from build123d import *

# Parameters (mm, degrees)
WALL_DEPTH                = 19.05
ROOF_START                = 19.05
ROOF_DEPTH                = 3.175
F_2_56_TAPPED_HOLE1_D     = 1.778
F_2_56_TAPPED_HOLE1_DEPTH = 5.73
F_2_56_TAPPED_HOLE1_TIP   = 0.53416509


with BuildPart() as part:
    # MainSketch → Wall (new body)
    with BuildSketch(Plane(origin=(0, 0, 0), x_dir=(1, 0, 0), z_dir=(0, 1, 0))):
        Polygon((-32.75, -4), (0, -4), (0, 0), (-36.75, 0), (-36.75, -45.5), (0, -45.5), (0, -41.5), (-32.75, -41.5), align=None)
    extrude(amount=WALL_DEPTH)

    # MainSketch<3> → Roof (add)
    with BuildSketch(Plane(origin=(0, 0, 0), x_dir=(1, 0, 0), z_dir=(0, 1, 0)).offset(ROOF_START)):
        with BuildLine():
            Line((0, -21.625), (0, 0))
            Line((0, 0), (-36.75, 0))
            Line((-36.75, 0), (-36.75, -45.5))
            Line((-36.75, -45.5), (0, -45.5))
            Line((0, -45.5), (0, -23.875))
            ThreePointArc((0, -23.875), (-0.353553391, -23.728553391), (-0.5, -23.375))
            Line((-0.5, -23.375), (-0.5, -22.125))
            ThreePointArc((-0.5, -22.125), (-0.353553391, -21.771446609), (0, -21.625))
        make_face()
    extrude(amount=ROOF_DEPTH)

    # #2-56 Tapped Hole1
    with Locations(Plane(origin=(-10, 0, 43), x_dir=(0, 0, -1), z_dir=(0, -1, 0))):
        with Locations((0, 0), (0, -24.25), (40.5, -24.25), (40.5, 0)):
            Hole(F_2_56_TAPPED_HOLE1_D / 2, depth=F_2_56_TAPPED_HOLE1_DEPTH)
            with Locations((0, 0, -(F_2_56_TAPPED_HOLE1_DEPTH + F_2_56_TAPPED_HOLE1_TIP / 2))):  # 118° drill point
                Cone(0, F_2_56_TAPPED_HOLE1_D / 2, F_2_56_TAPPED_HOLE1_TIP, mode=Mode.SUBTRACT)


solid = part.part
The listing builds one solid part. Answer for the finished solid, in the listing's coordinates (mm). A direction names the side the tool comes from. Round coordinates to 2 decimals unless told otherwise and drop trailing zeros. Order: outer loops, then holes, each group sorted by start corner. A loop starts at its lowest first (then second) coordinate and runs counter-clockwise, first axis right, second up. Notation, with made-up numbers: M 71.5,79.25 L 102.5,79.25 A33 ccw 102.5,117.25 Z; hole C 26.5,56.5 d4. An arc over 180 degrees is marked long. Answer in a Markdown table with one row per item. Add a question column.
1) The part is cut by section D-D on z = 20. Determine the outline of the cut face in (x, y) (3 decimals), plus the area to 3 significant figures.
2) Which of the six approach directions +Z, -Z, +X, -X, +Y, -Y give full straight-line access (tool end or side, diameter ignored) to faces 1 (the face through (-17, 19.05, 22)), 2 (the face through (-9.12, 2.91, 2.38)), 3 (the face through (-18, 11, 0))?
3) Consider line 1 along Z through (x, y) = (-10, 2.1); line 2 along X through (y, z) = (2.2, 43); line 3 along Z through (x, y) = (-34.25, 4). Determine where each line is inside the solid, lowest interval first. Write a range as from..to.
4) The part is cut by section B-B on x = -20. Determine the outline of the cut face in (y, z) (3 decimals).
5) The part is cut by section A-A on y = 3. Determine the outline of the cut face in (x, z), plus the area to 3 significant figures.
6) Flat-ended cylindrical pins translate along their axes: pin 1 Ø1.6 at (x, z) = (-34.25, 2.5) entering from -Y; pin 2 Ø0.6 at (y, z) = (20.5, 22.5) entering from +X; pin 3 Ø6 at (y, z) = (4, 14) entering from +X. Find the tip coordinate at first contact, or state that the pin passes through.
7) Determine the mould class of faces 4 (the face through (0, 14.4, 3.7)), 5 (the face through (-9.847, 6.171, 2.52)), 6 (the face through (-33, 0, 23)) for opening direction X: pulls with the +X half, pulls with the -X half, needs draft (parallel to the pull), parting line crosses it, or undercut.
8) The part is cut by section C-C on y = 12.25. Determine the outline of the cut face in (x, z), plus the area to 3 significant figures.
Findings below:
| question | item | result |
|---|---|---|
| 1 | outline | M -36.75,0 L -32.75,0 L -32.75,19.05 L 0,19.05 L 0,22.225 L -36.75,22.225 Z |
| 1 | area | 193 mm² |
| 2 | face 1 | +X, -Y |
| 2 | face 2 | -Y |
| 2 | face 3 | -Z, +X, -X, +Y, -Y |
| 3 | line 1 | z = 0..1.61, 3.39..4, 41.5..42.11, 43.89..45.5 |
| 3 | line 2 | x = -36.75..-35.14, -33.36..-10.89, -9.11..0 |
| 3 | line 3 | z = 0..1.61, 3.39..42.11, 43.89..45.5 |
| 4 | outline | M 0,0 L 22.225,0 L 22.225,45.5 L 0,45.5 L 0,41.5 L 19.05,41.5 L 19.05,4 L 0,4 Z |
| 5 | outline | M -36.75,0 L 0,0 L 0,4 L -32.75,4 L -32.75,41.5 L 0,41.5 L 0,45.5 L -36.75,45.5 Z; hole C -34.25,2.5 d1.78; hole C -34.25,43 d1.78; hole C -10,2.5 d1.78; hole C -10,43 d1.78 |
| 5 | area | 434 mm² |
| 6 | pin 1 | stops at y = 5.78 |
| 6 | pin 2 | stops at x = -0.5 |
| 6 | pin 3 | stops at x = -32.75 |
| 7 | face 4 | pulls with the +X half |
| 7 | face 5 | undercut |
| 7 | face 6 | needs draft |
| 8 | outline | M -36.75,0 L 0,0 L 0,4 L -32.75,4 L -32.75,41.5 L 0,41.5 L 0,45.5 L -36.75,45.5 Z |
| 8 | area | 444 mm² |
